```python
from build123d import *

# Parameters (mm, degrees)
BOSS_EXTRU_1_DEPTH                                 = 5
CONG_1_R                                           = 4
ENL_V_MAT_EXTRU_1_DEPTH                            = 10
ESQUISSE5_R                                        = 10.5
ENL_V_MAT_EXTRU_3_DEPTH                            = 3
CHAMBRAGE_POUR_VIS_T_TE_HEXAGONALE_M31_D           = 3.4
CHAMBRAGE_POUR_VIS_T_TE_HEXAGONALE_M31_CBORE_D     = 6.5
CHAMBRAGE_POUR_VIS_T_TE_HEXAGONALE_M31_CBORE_DEPTH = 3.4


with BuildPart() as part:
    # Esquisse1 → Boss.-Extru.1 (new body)
    with BuildSketch(Plane.XY):
        Polygon((-29.976777828, -25.077617952), (17.823222172, -25.077617952), (37.823222172, -5.077617952), (37.823222172, 7.922382048), (-30.176777828, 7.922382048), (-40.176777828, 7.922382048), (-40.176777828, -12.077617952), (-29.976777828, -12.077617952), align=None)
    extrude(amount=BOSS_EXTRU_1_DEPTH)

    # Congé1
    cong_1_edges = [part.edges().sort_by_distance(p)[0] for p in [
        (-29.976777828, -12.077617952, 2.5),
        (-40.176777828, -12.077617952, 2.5),
        (-40.176777828, 7.922382048, 2.5),
        (37.823222172, 7.922382048, 2.5),
        (37.823222172, -5.077617952, 2.5),
        (17.823222172, -25.077617952, 2.5),
        (-29.976777828, -25.077617952, 2.5),
    ]]
    fillet(cong_1_edges, radius=CONG_1_R)

    # Esquisse2 → Enlèv. mat.-Extru.1 (cut)
    with BuildSketch(Plane.XY.offset(5)):
        with BuildLine():
            Line((-5.470711646, 3.322382048), (1.117155991, 3.322382048))
            ThreePointArc((1.117155991, 3.322382048), (5.923222172, -4.077617952), (1.117155991, -11.477617952))
            Line((1.117155991, -11.477617952), (-5.470711646, -11.477617952))
            ThreePointArc((-5.470711646, -11.477617952), (-10.276777828, -4.077617952), (-5.470711646, 3.322382048))
        make_face()
        with BuildLine():
            Line((16.529288354, 3.322382048), (23.117155991, 3.322382048))
            ThreePointArc((23.117155991, 3.322382048), (27.923222172, -4.077617952), (23.117155991, -11.477617952))
            Line((23.117155991, -11.477617952), (16.529288354, -11.477617952))
            ThreePointArc((16.529288354, -11.477617952), (11.723222172, -4.077617952), (16.529288354, 3.322382048))
        make_face()
        with BuildLine():
            Line((-27.470711646, 3.322382048), (-20.882844009, 3.322382048))
            ThreePointArc((-20.882844009, 3.322382048), (-16.076777828, -4.077617952), (-20.882844009, -11.477617952))
            Line((-20.882844009, -11.477617952), (-27.470711646, -11.477617952))
            ThreePointArc((-27.470711646, -11.477617952), (-32.276777828, -4.077617952), (-27.470711646, 3.322382048))
        make_face()
    extrude(amount=-ENL_V_MAT_EXTRU_1_DEPTH, mode=Mode.SUBTRACT)

    # Esquisse5 → Enlèv. mat.-Extru.3 (cut)
    with BuildSketch(Plane.XY.offset(5)):
        with Locations((19.823222172, -4.077617952)):
            Circle(ESQUISSE5_R)
        with Locations((-2.176777828, -4.077617952)):
            Circle(ESQUISSE5_R)
        with Locations((-24.176777828, -4.077617952)):
            Circle(ESQUISSE5_R)
    extrude(amount=-ENL_V_MAT_EXTRU_3_DEPTH, mode=Mode.SUBTRACT)

    # Chambrage pour vis à tête hexagonale M31 (through all)
    with Locations(Plane.XY.offset(5)):
        with Locations((34.323222172, 1.922382048), (-11.976777828, -18.577617952)):
            CounterBoreHole(CHAMBRAGE_POUR_VIS_T_TE_HEXAGONALE_M31_D / 2, CHAMBRAGE_POUR_VIS_T_TE_HEXAGONALE_M31_CBORE_D / 2, CHAMBRAGE_POUR_VIS_T_TE_HEXAGONALE_M31_CBORE_DEPTH)


solid = part.part
```
Design review of the part built by this model. Coordinates are the model's own, in mm. A direction names the side the tool comes from. Round coordinates to 2 decimals unless told otherwise and drop trailing zeros. Write each loop counter-clockwise with the first axis right and the second up, starting at its lowest first coordinate (ties: lowest second). Pieces come first, ordered by that corner, then holes.
Item 1: Clearance check with flat-ended pins moving along their axes: pin 1 Ø5 at (x, y) = (-11.98, -18.58) entering from -Z; pin 2 Ø0.6 at (x, z) = (18.5, 0.5) entering from -Y; pin 3 Ø3 at (x, y) = (-11.5, -19.5) entering from +Z. State where each tip first meets the part, or that it passes through.
Item 2: We need section C-C on y = -0.5. State how many separate pieces and enclosed holes the cut face has, and give its area (3 significant figures).
Item 3: We need section B-B on y = -19.5. Write out the cut boundary in (x, z), and give its area (3 significant figures).
Item 4: For faces 5 (the flat face through (-24, -12, 2)), 6 (the flat face through (-29.977, -19, 2)), 7 (the flat face through (-2, -11.478, 1)), list the 3-axis set-ups (+Z, -Z, +X, -X, +Y, -Y) from which the entire face can be reached by the end or side of a thin tool; tool diameter is ignored.
Item 5: We need section A-A on x = 27. Write out the cut boundary in (y, z), and give its area (3 significant figures).
Item 6: For probe 1 along X at (y, z) = (-11, 3.75); probe 2 along X at (y, z) = (-1, 3.8); probe 3 along X at (y, z) = (-9.5, 3.9), list the stretches that pass through material, from the lowest coordinate up.
Item 7: The part is to be moulded in two halves that separate along Y. For faces 1 (the cylindrical face through (35.58, 3.07, 0.79)), 2 (the flat face through (36, 1, 1.6)), 3 (the flat face through (-35, -12.078, 2)), 4 (the flat face through (-10, -12, 5)), say which applies: +Y half, -Y half, draft (parallel to the pull), parting line (faces both ways), or undercut.
Item 8: We need section D-D on x = 11. Write out the cut boundary in (y, z).
Returned:
1. pin 1: stops at z = 0
1. pin 2: stops at y = -24.52
1. pin 3: stops at z = 1.6
2. separate pieces: 4
2. enclosed holes: 0
2. area: 110 mm2
3. outline: (-29.98, 0) - (-13.4, 0) - (-13.4, 1.6) - (-15.09, 1.6) - (-15.09, 5) - (-29.98, 5) - close; (-10.55, 0) - (23.4, 0) - (23.4, 5) - (-8.86, 5) - (-8.86, 1.6) - (-10.55, 1.6) - close
3. area: 241 mm2
4. face 5: +Z
4. face 6: +Z, -Z, -X, -Y
4. face 7: +Z, -Z
5. outline: (-15.9, 0) - (-7.83, 0) - (-7.83, 2) - (-11.74, 2) - (-11.74, 5) - (-15.9, 5) - close; (-0.32, 0) - (7.92, 0) - (7.92, 5) - (3.59, 5) - (3.59, 2) - (-0.32, 2) - close
5. area: 58.1 mm2
6. probe 1: x = -38.91 to -32.07, -16.28 to -10.07, 5.72 to 11.93, 27.72 to 31.9
6. probe 2: x = -40.18 to -34.22, -14.14 to -12.22, 7.86 to 9.78, 29.86 to 32.9, 35.75 to 37.82
6. probe 3: x = -39.92 to -33.17, -15.19 to -11.17, 6.81 to 10.83, 28.81 to 33.4
7. face 1: undercut
7. face 2: undercut
7. face 3: -Y half
7. face 4: draft
8. outline: (-25.08, 0) - (7.92, 0) - (7.92, 5) - (1.61, 5) - (1.61, 2) - (-9.77, 2) - (-9.77, 5) - (-25.08, 5) - close
